```python
from build123d import *

# Parameters (mm, degrees)
SKETCH1_W           = 120
SKETCH1_H           = 90
SKETCH1_R           = 1.5
BOSS_EXTRUDE1_DEPTH = 3
CHAMFER1_SIZE       = 1.5


with BuildPart() as part:
    # Sketch1 → Boss-Extrude1 (new body)
    with BuildSketch(Plane(origin=(0, 0, 0), x_dir=(1, 0, 0), z_dir=(0, 1, 0))):
        Rectangle(SKETCH1_W, SKETCH1_H)
        with Locations(Location((-55, 40, 0), (0, 0, 270))):
            Circle(SKETCH1_R, mode=Mode.SUBTRACT)
        with Locations(Location((-55, -40, 0), (0, 0, 270))):
            Circle(SKETCH1_R, mode=Mode.SUBTRACT)
        with Locations(Location((55, -40, 0), (0, 0, 270))):
            Circle(SKETCH1_R, mode=Mode.SUBTRACT)
        with Locations(Location((55, 40, 0), (0, 0, 270))):
            Circle(SKETCH1_R, mode=Mode.SUBTRACT)
    extrude(amount=BOSS_EXTRUDE1_DEPTH)

    # Chamfer1
    chamfer1_edges = [part.edges().sort_by_distance(p)[0] for p in [
        (-55, 3, -41.5),
        (-55, 3, 38.5),
        (55, 3, 38.5),
        (55, 3, -41.5),
    ]]
    chamfer(chamfer1_edges, length=CHAMFER1_SIZE)


solid = part.part
```
Read the model definition and answer for the solid it produces. Units are mm, in the model's axes. Give positions to 0.01 mm unless a question says otherwise; leave off trailing zeros. Write each loop counter-clockwise with the first axis right and the second up, starting at its lowest first coordinate (ties: lowest second). Pieces come first, ordered by that corner, then holes. Notation, with made-up numbers: (25.25, 46.5) - (61.25, 46.5) arc R9 cw to (61.25, 57.5) - close; hole circle Ø8 at (37, 39.25). An arc over 180 degrees is marked (long way). Write item = value, one per line. Start each with the question number.
Item 1: Each of these flat-tipped pins is pushed along its axis until it touches: P1, Ø2.5, axis at x = -55, z = -40, coming from the -Y side; P2, Ø4, axis at x = 55, z = -40, coming from the +Y side. Where does it stop, or does it pass through?
Item 2: Find section A-A (x = -55). Give the vertices of the cut face in (y, z).
Item 3: The mould has two halves that part along Z. Classify faces 1 (the cylindrical face through (54.1, 0.7, -41.2)), 2 (the flat face through (-60, 1, 1)), 3 (the flat face through (-1, 1, -45)), 4 (the flat face through (-1, 1, 45)): +Z half, -Z half, draft (parallel to the pull), parting line (faces both ways), or undercut.
Item 4: Find section B-B (z = -40). Give the vertices of the cut face in (x, y).
Item 5: Find the intervals of material crossed by probe 1 along X at (y, z) = (0.8, 40), in increasing order. Write a range as [from, to].
Response:
q1.P1 = through
q1.P2 = 2
q2.outline = (0, -45) - (3, -45) - (3, -43) - (1.5, -41.5) - (0, -41.5) - close; (0, -38.5) - (1.5, -38.5) - (3, -37) - (3, 37) - (1.5, 38.5) - (0, 38.5) - close; (0, 41.5) - (1.5, 41.5) - (3, 43) - (3, 45) - (0, 45) - close
q3.face_1 = undercut
q3.face_2 = draft
q3.face_3 = -Z half
q3.face_4 = +Z half
q4.outline = (-60, 0) - (-56.5, 0) - (-56.5, 1.5) - (-58, 3) - (-60, 3) - close; (-53.5, 0) - (53.5, 0) - (53.5, 1.5) - (52, 3) - (-52, 3) - (-53.5, 1.5) - close; (56.5, 0) - (60, 0) - (60, 3) - (58, 3) - (56.5, 1.5) - close
q5.probe_1 = [-60, -56.5], [-53.5, 53.5], [56.5, 60]
